The drawing under review shows one solid part. Ordinate dimensions are in mm from its lowest x, y, z. Give positions to 0.01 mm unless a question says otherwise; leave off trailing zeros. Order: outer loops, then holes, each group sorted by start corner. A loop starts at its lowest first (then second) coordinate and runs counter-clockwise, first axis right, second up. Notation, with made-up numbers: (5, 56.25) -> (21, 56.25) arc R33 ccw to (21, 85.25) -> close; hole circle Ø7 at (-39.75, 49.25). An arc over 180 degrees is marked (long way). Use a Markdown table: item, result. Add a question column.
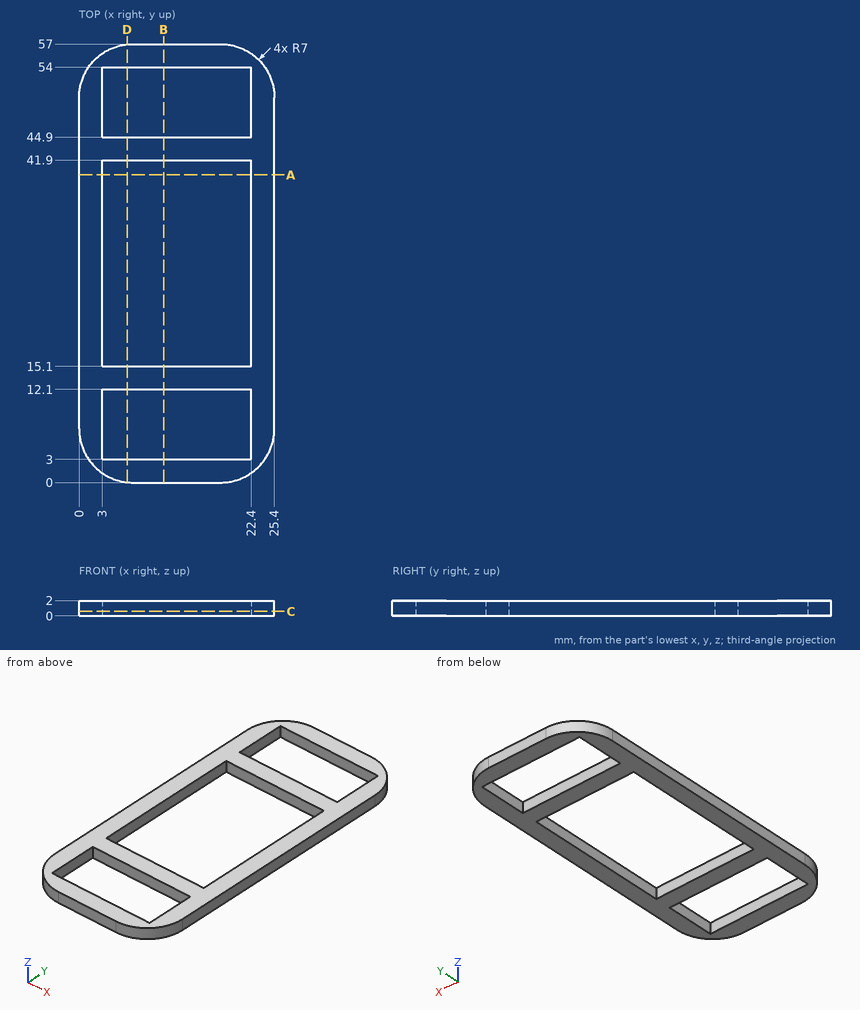
1) Add section D-D (x = 6.25). Give the boundary of the cut face in (y, z), then the cut area to 3 significant figures.
2) Add section A-A (y = 40). Give the boundary of the cut face in (x, z), then the cut area to 3 significant figures.
3) For L1, parallel to Y at x = 11.5, z = 1.4; L2, parallel to X at y = 8.5, z = 1.5; L3, parallel to Y at x = 6, z = 0.6, list the stretches that pass through material, from the lowest coordinate up. Write a range as [from, to].
4) Insertion check: pin 1 (4 mm diameter, centred on x = 17, y = 17.5, fed in from +Z); pin 2 (0.6 mm diameter, centred on y = 6, z = 1, fed in from -X). Each pin has a flat end and moves straight along its axis. Give the tip position at first contact, or say it passes through.
5) Add section C-C (z = 0.6). Give the boundary of the cut face in (x, y).
6) Add section B-B (x = 11). Give the boundary of the cut face in (y, z), then the cut area to 3 significant figures.
Worked answers:
| question | item | result |
|---|---|---|
| 1 | outline | (0.04, 0) -> (3, 0) -> (3, 2) -> (0.04, 2) -> close; (12.1, 0) -> (15.1, 0) -> (15.1, 2) -> (12.1, 2) -> close; (41.9, 0) -> (44.9, 0) -> (44.9, 2) -> (41.9, 2) -> close; (54, 0) -> (56.96, 0) -> (56.96, 2) -> (54, 2) -> close |
| 1 | area | 23.8 mm^2 |
| 2 | outline | (0, 0) -> (3, 0) -> (3, 2) -> (0, 2) -> close; (22.4, 0) -> (25.4, 0) -> (25.4, 2) -> (22.4, 2) -> close |
| 2 | area | 12.0 mm^2 |
| 3 | L1 | [0, 3], [12.1, 15.1], [41.9, 44.9], [54, 57] |
| 3 | L2 | [0, 3], [22.4, 25.4] |
| 3 | L3 | [0.07, 3], [12.1, 15.1], [41.9, 44.9], [54, 56.93] |
| 4 | pin 1 | through |
| 4 | pin 2 | x = 0.04 |
| 5 | outline | (0, 7) arc R7 ccw to (7, 0) -> (18.4, 0) arc R7 ccw to (25.4, 7) -> (25.4, 50) arc R7 ccw to (18.4, 57) -> (7, 57) arc R7 ccw to (0, 50) -> close; hole (3, 3) -> (22.4, 3) -> (22.4, 12.1) -> (3, 12.1) -> close; hole (3, 15.1) -> (22.4, 15.1) -> (22.4, 41.9) -> (3, 41.9) -> close; hole (3, 44.9) -> (22.4, 44.9) -> (22.4, 54) -> (3, 54) -> close |
| 6 | outline | (0, 0) -> (3, 0) -> (3, 2) -> (0, 2) -> close; (12.1, 0) -> (15.1, 0) -> (15.1, 2) -> (12.1, 2) -> close; (41.9, 0) -> (44.9, 0) -> (44.9, 2) -> (41.9, 2) -> close; (54, 0) -> (57, 0) -> (57, 2) -> (54, 2) -> close |
| 6 | area | 24.0 mm^2 |
